from build123d import *

# Parameters (mm, degrees)
F0_R     = 4.572
F1_DEPTH = 76.2
F3_DEPTH = 2.54
F5_DEPTH = 2.54


with BuildPart() as f1:
    # F0 (on Front) → F1 (new body)
    with BuildSketch(Plane.XZ):
        Circle(F0_R)
    extrude(amount=F1_DEPTH)

    # F2 (on face) → F3 (cut)
    with BuildSketch(Plane.XZ.offset(76.2)):
        with BuildLine():
            Line((1.9650808536, 8.0974539742), (-1.5526660718, 8.0974539742))
            Line((-1.5526660718, 8.0974539742), (-1.5526660718, 4.300280464))
            ThreePointArc((-1.5526660718, 4.300280464), (0.2234468976, 4.5665364867), (1.9650808536, 4.128152279))
            Line((1.9650808536, 4.128152279), (1.9650808536, 8.0974539742))
        make_face()
        with BuildLine():
            ThreePointArc((1.9650808536, -4.128152279), (0.2234468976, -4.5665364867), (-1.5526660718, -4.300280464))
            Line((-1.5526660718, -4.300280464), (-1.5526660718, -7.655933965))
            Line((-1.5526660718, -7.655933965), (1.9650808536, -7.655933965))
            Line((1.9650808536, -7.655933965), (1.9650808536, -4.128152279))
        make_face()
        with BuildLine():
            ThreePointArc((1.9650808536, 4.128152279), (0.2234468976, 4.5665364867), (-1.5526660718, 4.300280464))
            Line((-1.5526660718, 4.300280464), (-1.5526660718, -4.300280464))
            ThreePointArc((-1.5526660718, -4.300280464), (0.2234468976, -4.5665364867), (1.9650808536, -4.128152279))
            Line((1.9650808536, -4.128152279), (1.9650808536, 4.128152279))
        make_face()
    extrude(amount=-F3_DEPTH, mode=Mode.SUBTRACT)

    # F4 (on face) → F5 (cut)
    with BuildSketch(Plane(origin=(0, 0, 0), x_dir=(-1, 0, 0), z_dir=(0, 1, 0))):
        with BuildLine():
            ThreePointArc((1.6067995457, 4.2803480256), (0.082074117, 4.5712632652), (-1.4521116391, 4.3352688253))
            Line((-1.4521116391, 4.3352688253), (-1.4521116391, -4.3352688253))
            ThreePointArc((-1.4521116391, -4.3352688253), (0.082074117, -4.5712632652), (1.6067995457, -4.2803480256))
            Line((1.6067995457, -4.2803480256), (1.6067995457, 4.2803480256))
        make_face()
    extrude(amount=-F5_DEPTH, mode=Mode.SUBTRACT)


solid = f1.part
Geometry: final body of the model. Coordinates: model frame, mm. A direction names the side the tool comes from. Coordinates: 2 decimals unless noted, no trailing zeros. Order: outer loops, then holes, each group sorted by start corner. A loop starts at its lowest first (then second) coordinate and runs counter-clockwise, first axis right, second up. Notation, with made-up numbers: (46.5, 72.5) - (52.5, 72.5) arc R8 ccw to (52.5, 83.5) - close; hole circle Ø10 at (-36, 14). An arc over 180 degrees is marked (long way). Use one line per item in the form item = value.
1) Section A-A (z = 0). Return loops of the section in (x, y), then the cut area to 3 significant figures.
Solutions:
outline = (-4.57, -76.2) - (-1.55, -76.2) - (-1.55, -73.66) - (1.97, -73.66) - (1.97, -76.2) - (4.57, -76.2) - (4.57, 0) - (1.45, 0) - (1.45, -2.54) - (-1.61, -2.54) - (-1.61, 0) - (-4.57, 0) - close
area = 680 mm^2
2) Section B-B (y = -23). Return loops of the section in (x, z), then the cut area to 3 significant figures.
Solutions:
outline = circle Ø9.14 at (0, 0)
area = 65.7 mm^2
3) Mould query, pull axis X, two halves, no side actions, for faces 1 (the face through (3, -76.2, 0)), 2 (the face through (-0.991, -37.567, -4.463)), 3 (the face through (-1.553, -75, 0)). Classes: +X half, -X half, draft (parallel to the pull), parting line (faces both ways), or undercut.
Solutions:
face_1 = draft
face_2 = parting line
face_3 = undercut
4) Pin query (flat end, axial travel): pin 1 (0.8 mm diameter, centred on y = -75, z = 1, fed in from -X); pin 2 (5 mm diameter, centred on y = -23, z = 3.5, fed in from +X); pin 3 (0.9 mm diameter, centred on x = 0, z = -2, fed in from +Y); pin 4 (1 mm diameter, centred on x = -1.5, z = 3, fed in from -Y). Return the tip coordinate at first contact, or that it passes through.
Solutions:
pin_1 = -4.53
pin_2 = 4.46
pin_3 = -2.54
pin_4 = -76.2
5) Ray query, L1, parallel to Y at x = 1.75, z = 2; L2, parallel to Y at x = -1.25, z = 3.5; L3, parallel to X at y = -52, z = -0.25. Return the intervals inside material, ascending.
Solutions:
L1 = -73.66 to 0
L2 = -73.66 to -2.54
L3 = -4.57 to 4.57
6) Set-up query: faces 4 (the face through (0, -73.66, 0)), 5 (the face through (-3, 0, 0)), 6 (the face through (-1.607, -1, 0)). Return all of +Z, -Z, +X, -X, +Y, -Y with unobstructed straight access to the full face (end or side cutting, diameter ignored); none if empty.
Solutions:
face_4 = +Z, -Z, -Y
face_5 = +Z, -Z, +X, -X, +Y
face_6 = +Z, -Z, +Y
7) Section C-C (x = 0). Return loops of the section in (y, z).
Solutions:
outline = (-73.66, -4.57) - (-2.54, -4.57) - (-2.54, 4.57) - (-73.66, 4.57) - close
